Could you check a few things on this model? Use its own coordinates, in mm. A direction names the side the tool comes from. Round coordinates to 2 decimals unless told otherwise and drop trailing zeros. Order: outer loops, then holes, each group sorted by start corner. A loop starts at its lowest first (then second) coordinate and runs counter-clockwise, first axis right, second up. Notation, with made-up numbers: M 51,1 L 55,1 A31 cw 55,36 Z; hole C -21.75,42 d11. An arc over 180 degrees is marked long. Write each question's results on one line, items separated by ' | '. Start each with the question number.
1. Suppose I cut it at A-A on y = 1.5. Write out the boundary of the cut face in (x, z), and give its area (3 significant figures).
2. I'm going to push flat-ended pins straight in: pin 1 (5 mm diameter, centred on x = -17.5, y = 22.5, fed in from -Z); pin 2 (1 mm diameter, centred on y = 11.5, z = 10, fed in from -X); pin 3 (2 mm diameter, centred on y = 13.5, z = -21, fed in from +X). Where does each tip first touch, or does it pass through?
3. We'd pull the mould along Y, two halves only. Please class faces 4 (the flat face through (-21.5, -18.52, -15.23)), 5 (the flat face through (-25, -17, -13)): released by +Y, released by -Y, zero draft, split by the parting line, or undercut.
4. Please list where these lines run through material, in increasing order: L1, parallel to Y at x = -1, z = 26; L2, parallel to Y at x = -11, z = -6; L3, parallel to X at y = -4, z = 25.5.
5. Suppose I cut it at B-B on x = -22. Write out the boundary of the cut face in (y, z), and give its area (3 significant figures).
6. For faces 1 (the cylindrical face through (-10.07, 7.34, 1.76)), 2 (the flat face through (8.086, -10.14, 32.049)), 3 (the flat face through (-8.046, 6.902, 7.131)), which set-ups out of +Z, -Z, +X, -X, +Y, -Y let a thin tool reach every point of the face, with its end or its side?
7. Suppose I cut it at C-C on z = -6. Write out the boundary of the cut face in (x, y), and give its area (3 significant figures).
8. Suppose I cut it at D-D on y = 19.5. Write out the boundary of the cut face in (x, z).
from build123d import *

# Parameters (mm, degrees)
BOSS_EXTRUDE1_DEPTH      = 14
SKETCH3_R                = 4.125
CUT_EXTRUDE1_DEPTH       = 6
SKETCH5_R                = 1.125
CUT_EXTRUDE2_DEPTH       = 15
FILLET1_R                = 1
BOSS_EXTRUDE3_DEPTH      = 20
BOSS_EXTRUDE3_DEPTH_BACK = 34
SKETCH7_W                = 46.707438453
SKETCH7_H                = 20
CUT_EXTRUDE3_DEPTH       = 30
BOSS_EXTRUDE4_DEPTH      = 3
BOSS_EXTRUDE5_START      = -54
BOSS_EXTRUDE5_DEPTH      = 3
CUT_EXTRUDE5_REACH       = 111.564
SKETCH15_W               = 26.880557743
SKETCH15_H               = 40.856784115
CUT_EXTRUDE6_REACH       = 113.249
SKETCH16_R               = 1.6
CUT_EXTRUDE7_DEPTH       = 108.082055537
CUT_EXTRUDE7_DEPTH_BACK  = 108.082055537
SKETCH19_W               = 109.652108874
SKETCH19_H               = 14
SKETCH21_W               = 96.727229551
SKETCH21_H               = 14
CUT_EXTRUDE8_DEPTH       = 79.38857666
SKETCH22_R               = 2.6
CUT_EXTRUDE9_DEPTH       = 83.047416404


with BuildPart() as part:
    # Sketch1 → Boss-Extrude1 (new body)
    with BuildSketch(Plane(origin=(0, 0, 0), x_dir=(1, 0, 0), z_dir=(0, 1, 0))):
        with BuildLine():
            Line((47.5, -78.442713945), (47.5, -38.442713945))
            ThreePointArc((47.5, -38.442713945), (23.122023742, 0), (47.5, 38.442713945))
            Line((47.5, 38.442713945), (47.5, 50))
            Line((47.5, 50), (42.5, 50))
            Line((42.5, 50), (0, 0))
            Line((0, 0), (35.1, -73.422380253))
            Line((35.1, -73.422380253), (35.1, -93.442713945))
            Line((35.1, -93.442713945), (37.5, -93.442713945))
            Line((37.5, -93.442713945), (47.5, -93.442713945))
            Line((47.5, -93.442713945), (47.5, -78.442713945))
        make_face()
    extrude(amount=BOSS_EXTRUDE1_DEPTH)

    # Sketch3 → Cut-Extrude1 (cut)
    with BuildSketch(Plane.XZ):
        with BuildLine():
            Line((33.254958794, 84.403112572), (36.18509612, 92.428977457))
            Line((36.18509612, 92.428977457), (44.88509612, 92.428977457))
            Line((44.88509612, 92.428977457), (46.13509612, 88.028977457))
            Line((46.13509612, 88.028977457), (46.13509612, 70.028977457))
            Line((46.13509612, 70.028977457), (44.820911197, 53.062159312))
            ThreePointArc((44.820911197, 53.062159312), (40.059955227, 48.679043991), (35.34566343, 53.112310791))
            Line((35.34566343, 53.112310791), (33.254958794, 84.403112572))
        make_face()
        with Locations(Location((40.08509612, 83.428977457, 0), (0, 0, 90))):
            Circle(SKETCH3_R, mode=Mode.SUBTRACT)
    extrude(amount=-CUT_EXTRUDE1_DEPTH, mode=Mode.SUBTRACT)

    # Sketch5 → Cut-Extrude2 (cut)
    with BuildSketch(Plane.XZ.offset(-6)):
        with Locations(Location((40.08509612, 63.428977457, 0), (0, 0, 270))):
            Circle(SKETCH5_R)
        with Locations(Location((40.08509612, 58.928977457, 0), (0, 0, 270))):
            Circle(SKETCH5_R)
        with Locations(Location((40.08509612, 53.428977457, 0), (0, 0, 270))):
            Circle(SKETCH5_R)
    extrude(amount=-CUT_EXTRUDE2_DEPTH, mode=Mode.SUBTRACT)

    # Fillet1
    fillet1_edges = [part.edges().sort_by_distance(p)[0] for p in [
        (21.25, 0, -25),
        (45, 0, -50),
        (47.5, 0, -44.221356973),
        (23.122023742, 14, 0),
        (23.122023742, 0, 0),
        (47.5, 0, 65.942713945),
        (47.5, 14, -44.221356973),
        (42.5, 7, -50),
        (47.5, 7, -50),
        (47.5, 7, -38.442713945),
        (47.5, 7, 38.442713945),
        (45, 14, -50),
        (21.25, 14, -25),
        (47.5, 14, 65.942713945),
    ]]
    fillet(fillet1_edges, radius=FILLET1_R)

    # Sketch6 → Boss-Extrude3 (add, two sides: drawn at the far end of the back side and taken through both)
    with BuildSketch(Plane.XZ.offset(-BOSS_EXTRUDE3_DEPTH_BACK)):
        with BuildLine():
            Line((-40.458581161, -20.077158004), (-49.887563088, -23.407968691))
            Line((-49.887563088, -23.407968691), (34.124921356, 71.382705183))
            Line((34.124921356, 71.382705183), (0, 0))
            ThreePointArc((0, 0), (-10.212270894, 1.77453397), (-20.560220827, 2.374016932))
            Line((-20.560220827, 2.374016932), (-40.458581161, -20.077158004))
        make_face()
    extrude(amount=BOSS_EXTRUDE3_DEPTH + BOSS_EXTRUDE3_DEPTH_BACK)

    # Sketch7 → Cut-Extrude3 (cut)
    with BuildSketch(Plane(origin=(-16.32086192, 0, 14.465095586), x_dir=(0.6632786778078259, 0, 0.7483724978682089), z_dir=(-0.7483724978682089, 0, 0.6632786778078259))):
        with Locations((52.701466874, 24)):
            Rectangle(SKETCH7_W, SKETCH7_H)
        with Locations((52.701466874, -10)):
            Rectangle(SKETCH7_W, SKETCH7_H)
    extrude(amount=-CUT_EXTRUDE3_DEPTH, mode=Mode.SUBTRACT)

    # Sketch10 → Boss-Extrude4 (add)
    with BuildSketch(Plane.XZ.offset(20)):
        Polygon((-49.887563088, -23.407968691), (-42.403838109, -30.040755469), (0, 0), (-16.723629197, 14.010656202), align=None)
    extrude(amount=-BOSS_EXTRUDE4_DEPTH)

    # Sketch10<2> → Boss-Extrude5 (add)
    with BuildSketch(Plane.XZ.offset(20).offset(BOSS_EXTRUDE5_START)):
        Polygon((-49.887563088, -23.407968691), (-42.403838109, -30.040755469), (0, 0), (-16.723629197, 14.010656202), align=None)
    extrude(amount=BOSS_EXTRUDE5_DEPTH)

    # Cut-Extrude5: up to this face of the body (flat: up to its plane)
    cut_extrude5_end = Plane(part.part.faces().sort_by_distance((40.08509612, 0, 83.428977457))[0])
    # Sketch15 → Cut-Extrude5 (cut, up to the picked face)
    with BuildSketch(Plane(origin=(0, 6, 0), x_dir=(-1, 0, 0), z_dir=(0, -1, 0)), mode=Mode.PRIVATE) as cut_extrude5_sk1:
        with Locations((-44.420319758, -91.811097241)):
            Rectangle(SKETCH15_W, SKETCH15_H)
    cut_extrude5_tool1 = split(extrude(cut_extrude5_sk1.sketch, amount=CUT_EXTRUDE5_REACH, mode=Mode.PRIVATE), bisect_by=cut_extrude5_end, keep=Keep.BOTH, mode=Mode.PRIVATE)
    add(cut_extrude5_tool1.solids().sort_by(Axis((44.42032, 6, 91.811097), (0, -1, 0)))[0], mode=Mode.SUBTRACT)

    # Sketch16 → Cut-Extrude6 (cut, up to next)
    with BuildSketch(Plane(origin=(0, 14, 0), x_dir=(1, 0, 0), z_dir=(0, 1, 0)), mode=Mode.PRIVATE) as cut_extrude6_sk1:
        with Locations(Location((40.08509612, -83.428977457, 0), (0, 0, 270))):
            Circle(SKETCH16_R)
    cut_extrude6_tool1 = extrude(cut_extrude6_sk1.sketch, amount=-CUT_EXTRUDE6_REACH, mode=Mode.PRIVATE) & part.part
    add(cut_extrude6_tool1.solids().sort_by_distance((40.085096, 14, 83.428977))[0], mode=Mode.SUBTRACT)

    # Sketch19 → Cut-Extrude7 (cut, two sides: drawn at the far end of the back side and taken through both)
    with BuildSketch(Plane(origin=(-16.32086192, 0, 14.465095586), x_dir=(0.6632786778078262, 0, 0.7483724978682087), z_dir=(-0.7483724978682087, 0, 0.6632786778078262)).offset(-CUT_EXTRUDE7_DEPTH_BACK)):
        with Locations((54.826054437, 7)):
            Rectangle(SKETCH19_W, SKETCH19_H)
    extrude(amount=CUT_EXTRUDE7_DEPTH + CUT_EXTRUDE7_DEPTH_BACK, mode=Mode.SUBTRACT)


with BuildPart() as cut_extrude7_piece_1:
    # of the separate pieces the step leaves, piece 1, a body of its own (cut_extrude7_pieces)
    add(part.part.solids().sort_by_distance((3.144873335, 0, 36.428142799))[0])

    # Sketch22 → Cut-Extrude9 (cut, through all)
    with BuildSketch(Plane(origin=(0, -20, 0), x_dir=(-1, 0, 0), z_dir=(0, -1, 0))):
        with Locations(Location((5.733478103, -15.103299236, 0), (0, 0, 90))):
            Circle(SKETCH22_R)
        with Locations(Location((-4.215702064, -26.328886704, 0), (0, 0, 90))):
            Circle(SKETCH22_R)
    extrude(amount=-CUT_EXTRUDE9_DEPTH, mode=Mode.SUBTRACT)


with BuildPart() as cut_extrude7_piece_2:
    # of the separate pieces the step leaves, piece 2, a body of its own (cut_extrude7_pieces)
    add(part.part.solids().sort_by_distance((46.5, 0, -41.212709721))[0])

    # Sketch21 → Cut-Extrude8 (cut, through all)
    with BuildSketch(Plane(origin=(0, 0, 0), x_dir=(-0.4313049702307203, 0, -0.902206197415135), z_dir=(0.902206197415135, 0, -0.4313049702307203))):
        with Locations((24.708571423, 7)):
            Rectangle(SKETCH21_W, SKETCH21_H)
    extrude(amount=CUT_EXTRUDE8_DEPTH, mode=Mode.SUBTRACT)


solid = cut_extrude7_piece_1.part
Filled sheet:
1) outline: M -49.89,-23.41 L -40.46,-20.08 L -20.56,2.37 A90.83 cw 0,0 L -16.32,14.47 Z | area: 317 mm^2
2) pin 1: stops at z = 2.2 | pin 2: stops at x = -20.72 | pin 3: stops at x = -40.39
3) face 4: zero draft | face 5: undercut
4) L1: y = -20 to 0, 14 to 34 | L2: y = -20 to -17, 31 to 34 | L3: x = -6.54 to 1.75, 6.68 to 12.19
5) outline: M -20,-15.59 L -17,-15.59 L -17,0.75 L 31,0.75 L 31,-15.59 L 34,-15.59 L 34,8.06 L -20,8.06 Z | area: 493 mm^2
6) face 1: -Z | face 2: +Z, +X, +Y, -Y | face 3: +Z, +X
7) outline: M -34.46,-20 L -8.47,-20 L -8.47,-17 L -27.98,-17 L -27.98,31 L -8.47,31 L -8.47,34 L -34.46,34 Z | area: 467 mm^2
8) outline: M -49.89,-23.41 L -40.46,-20.08 L -20.56,2.37 A90.83 cw 0,0 L 13.17,27.54 L 3.14,36.43 Z; hole C -5.73,15.1 d5.2; hole C 4.22,26.33 d5.2
